For this review, take the finished solid that the model builds, in its own axes (mm). A direction names the side the tool comes from. Give positions to 0.01 mm unless a question says otherwise; leave off trailing zeros. Write each loop counter-clockwise with the first axis right and the second up, starting at its lowest first coordinate (ties: lowest second). Pieces come first, ordered by that corner, then holes. Notation, with made-up numbers: M 21.25,-3.75 L 61.25,-3.75 A10 ccw 61.25,10.25 Z; hole C 5.25,-8 d3. An arc over 180 degrees is marked long. One line per item, written item: value. Start each with the question number.
Item 1: Consider section D-D, the plane z = 29.5. Write out the cut boundary in (x, y).
Item 2: Mouldability with a two-part tool opening along X and no side actions: class faces 4 (the face through (-7.5, 21, 59)), 5 (the face through (-17.567, 23.768, -19.914)), 6 (the face through (25, 21, -25)) as released by +X, released by -X, zero draft, split by the parting line, or undercut.
Item 3: Consider section B-B, the plane z = 50. Write out the cut boundary in (x, y), and give its area (3 significant figures).
Item 4: Clearance check with flat-ended pins moving along their axes: pin 1 Ø1.5 at (y, z) = (23, -17) entering from -X; pin 2 Ø3 at (x, z) = (19.5, 18.5) entering from -Y; pin 3 Ø2 at (y, z) = (23, -42.5) entering from -X; pin 4 Ø5 at (x, z) = (50, 0) entering from -Y. State where each tip first meets the part, or that it passes through.
Item 5: Consider section C-C, the plane x = 0. Write out the cut boundary in (y, z) (3 decimals).
Item 6: Tool access review of faces 1 (the face through (7.5, 21, -59)), 2 (the face through (20.31, 22.5, -17.69)), 3 (the face through (-59, 21, -7.5)): name each direction out of +Z, -Z, +X, -X, +Y, -Y from which nothing blocks a thin tool from reaching the whole face with its end or side.
Item 7: To check wall thickness, follow probe 1 along X at (y, z) = (22, -50); probe 2 along Z at (x, y) = (0, 21); probe 3 along X at (y, z) = (23.6, -19). State the ranges of each line that lie inside material, in increasing order.
Item 8: Consider section A-A, the plane x = -50. Write out the cut boundary in (y, z), and give its area (3 significant figures).
```python
from build123d import *

# Parameters (mm, degrees)
SKETCH1_W               = 50
SKETCH1_H               = 50
BOSS_EXTRUDE1_DEPTH     = 25
CUT_EXTRUDE1_DEPTH      = 44.301270189
CUT_EXTRUDE1_DEPTH_BACK = 44.301270189
SKETCH3_R               = 5.1
CUT_EXTRUDE2_DEPTH      = 62.23724357
CUT_EXTRUDE2_DEPTH_BACK = 62.23724357
SKETCH4_W               = 50
SKETCH4_H               = 18
CUT_EXTRUDE3_START      = -2.5
SKETCH5_R               = 1.7
CUT_EXTRUDE3_DEPTH      = 34.541642582
CUT_EXTRUDE5_DEPTH      = 37.041642582
CUT_EXTRUDE5_DEPTH_BACK = 37.041642582
SKETCH6_R               = 1.7
BOSS_EXTRUDE5_DEPTH     = 7
SKETCH8_R               = 3.25
CUT_EXTRUDE6_DEPTH      = 107.296754419
CIRPATTERN1_COUNT       = 4


with BuildPart() as part:
    # Sketch1 → Boss-Extrude1 (new body)
    with BuildSketch(Plane(origin=(0, 0, 0), x_dir=(1, 0, 0), z_dir=(0, 1, 0))):
        Rectangle(SKETCH1_W, SKETCH1_H)
    extrude(amount=BOSS_EXTRUDE1_DEPTH)

    # Sketch2 → Cut-Revolve1 (revolve, cut)
    with BuildSketch(Plane.XY):
        with BuildLine():
            Line((-15.125, 25), (0, 25))
            Line((0, 25), (0, 9.875))
            ThreePointArc((0, 9.875), (-10.694990065, 14.305009935), (-15.125, 25))
        make_face()
    revolve(axis=Axis((0, 25, 0), (0, -1, 0)), mode=Mode.SUBTRACT)

    # Sketch3 → Cut-Extrude1 (cut, two sides: drawn at the far end of the back side and taken through both)
    with BuildSketch(Plane.XZ.offset(-CUT_EXTRUDE1_DEPTH_BACK)):
        with Locations(Location((0, 0, 0), (0, 0, 90))):
            Circle(SKETCH3_R)
    extrude(amount=CUT_EXTRUDE1_DEPTH + CUT_EXTRUDE1_DEPTH_BACK, mode=Mode.SUBTRACT)

    # Sketch4 → Cut-Extrude2 (cut, two sides: drawn at the far end of the back side and taken through both)
    with BuildSketch(Plane.ZY.offset(25).offset(-CUT_EXTRUDE2_DEPTH_BACK)):
        with Locations((0, 9)):
            Rectangle(SKETCH4_W, SKETCH4_H)
    extrude(amount=CUT_EXTRUDE2_DEPTH + CUT_EXTRUDE2_DEPTH_BACK, mode=Mode.SUBTRACT)

    # Sketch5 → Cut-Extrude3 (cut, through all)
    # profile 1 of 4: a face of its own
    with BuildSketch(Plane(origin=(0, 25, 0), x_dir=(1, 0, 0), z_dir=(0, 1, 0)).offset(CUT_EXTRUDE3_START)):
        Polygon((22.03934257, 19.814389387), (19.814389387, 22.03934257), (16.775046817, 21.224953183), (15.96065743, 18.185610613), (18.185610613, 15.96065743), (21.224953183, 16.775046817), align=None)
        with Locations(Location((19, 19, 0), (0, 0, 270))):
            Circle(SKETCH5_R, mode=Mode.SUBTRACT)
    # profile 2 of 4: a face of its own
    with BuildSketch(Plane(origin=(0, 25, 0), x_dir=(1, 0, 0), z_dir=(0, 1, 0)).offset(CUT_EXTRUDE3_START)):
        Polygon((-16.775046817, 21.224953183), (-19.814389387, 22.03934257), (-22.03934257, 19.814389387), (-21.224953183, 16.775046817), (-18.185610613, 15.96065743), (-15.96065743, 18.185610613), align=None)
        with Locations(Location((-19, 19, 0), (0, 0, 270))):
            Circle(SKETCH5_R, mode=Mode.SUBTRACT)
    # profile 3 of 4: a face of its own
    with BuildSketch(Plane(origin=(0, 25, 0), x_dir=(1, 0, 0), z_dir=(0, 1, 0)).offset(CUT_EXTRUDE3_START)):
        Polygon((19.814389387, -22.03934257), (22.03934257, -19.814389387), (21.224953183, -16.775046817), (18.185610613, -15.96065743), (15.96065743, -18.185610613), (16.775046817, -21.224953183), align=None)
        with Locations(Location((19, -19, 0), (0, 0, 270))):
            Circle(SKETCH5_R, mode=Mode.SUBTRACT)
    # profile 4 of 4: a face of its own
    with BuildSketch(Plane(origin=(0, 25, 0), x_dir=(1, 0, 0), z_dir=(0, 1, 0)).offset(CUT_EXTRUDE3_START)):
        Polygon((-22.03934257, -19.814389387), (-19.814389387, -22.03934257), (-16.775046817, -21.224953183), (-15.96065743, -18.185610613), (-18.185610613, -15.96065743), (-21.224953183, -16.775046817), align=None)
        with Locations(Location((-19, -19, 0), (0, 0, 270))):
            Circle(SKETCH5_R, mode=Mode.SUBTRACT)
    extrude(amount=-CUT_EXTRUDE3_DEPTH, mode=Mode.SUBTRACT)

    # Sketch6 → Cut-Extrude5 (cut, two sides: drawn at the far end of the back side and taken through both)
    with BuildSketch(Plane.XZ.offset(-18).offset(-CUT_EXTRUDE5_DEPTH_BACK)):
        with Locations(Location((-19, -19, 0), (0, 0, 270))):
            Circle(SKETCH6_R)
        with Locations(Location((19, -19, 0), (0, 0, 270))):
            Circle(SKETCH6_R)
        with Locations(Location((19, 19, 0), (0, 0, 270))):
            Circle(SKETCH6_R)
        with Locations(Location((-19, 19, 0), (0, 0, 270))):
            Circle(SKETCH6_R)
    extrude(amount=CUT_EXTRUDE5_DEPTH + CUT_EXTRUDE5_DEPTH_BACK, mode=Mode.SUBTRACT)

    # Sketch7 → Boss-Extrude5 (add)
    with BuildSketch(Plane.XZ.offset(-18)):
        Polygon((42.5, 7.5), (25, 25), (25, -25), (42.5, -7.5), (75, -7.5), (75, 7.5), align=None)
        Polygon((-25, 25), (25, 25), (7.5, 42.5), (7.5, 75), (-7.5, 75), (-7.5, 42.5), align=None)
        Polygon((7.5, -42.5), (25, -25), (-25, -25), (-7.5, -42.5), (-7.5, -75), (7.5, -75), align=None)
        Polygon((-25, -25), (-25, 25), (-42.5, 7.5), (-75, 7.5), (-75, -7.5), (-42.5, -7.5), align=None)
    extrude(amount=-BOSS_EXTRUDE5_DEPTH)

    # Sketch8 → Cut-Extrude6 (cut, symmetric)
    with BuildSketch(Plane.XZ.offset(-18)):
        with Locations(Location((50, 0, 0), (0, 0, 270))):
            Circle(SKETCH8_R)
    cut_extrude6 = extrude(amount=CUT_EXTRUDE6_DEPTH, both=True, mode=Mode.SUBTRACT)

    # CirPattern1: Cut-Extrude6 ×4 about axis
    cirpattern1_axis = Axis((0, 0, 0), (0, 1, 0))
    for i in range(1, CIRPATTERN1_COUNT):
        add(cut_extrude6.rotate(cirpattern1_axis, i * 360 / CIRPATTERN1_COUNT), mode=Mode.SUBTRACT)

    # Sketch2<2> → Cut-Revolve2 (revolve, cut)
    with BuildSketch(Plane.XY):
        with BuildLine():
            Line((-15.125, 25), (0, 25))
            Line((0, 25), (0, 9.875))
            ThreePointArc((0, 9.875), (-10.694990065, 14.305009935), (-15.125, 25))
        make_face()
    revolve(axis=Axis((0, 25, 0), (0, -1, 0)), mode=Mode.SUBTRACT)


solid = part.part
```
Model answer:
1. outline: M -20.5,18 L 20.5,18 L 20.5,25 L -20.5,25 Z
2. face 4: released by -X
2. face 5: undercut
2. face 6: released by +X
3. outline: M -7.5,18 L -3.25,18 L -3.25,25 L -7.5,25 Z; M 3.25,18 L 7.5,18 L 7.5,25 L 3.25,25 Z
3. area: 59.5 mm2
4. pin 1: stops at x = -33.75
4. pin 2: stops at y = 22.5
4. pin 3: stops at x = -8.5
4. pin 4: passes through
5. outline: M 18,-75 L 25,-75 L 25,-53.25 L 18,-53.25 Z; M 18,-46.75 L 25,-46.75 L 25,-15.125 A15.125 cw 18,-13.408 Z; M 18,13.408 A15.125 cw 25,15.125 L 25,46.75 L 18,46.75 Z; M 18,53.25 L 25,53.25 L 25,75 L 18,75 Z
6. face 1: -Z, +X, +Y, -Y
6. face 2: -Y
6. face 3: -Z, -X, +Y, -Y
7. probe 1: x = -7.5 to -3.25, 3.25 to 7.5
7. probe 2: z = -75 to -53.25, -46.75 to -14.59, 14.59 to 46.75, 53.25 to 75
7. probe 3: x = -31 to -20.7, -17.3 to 17.3, 20.7 to 31
8. outline: M 18,-7.5 L 25,-7.5 L 25,-3.25 L 18,-3.25 Z; M 18,3.25 L 25,3.25 L 25,7.5 L 18,7.5 Z
8. area: 59.5 mm2
